Build history of the part. All positions in model axes, mm. A direction names the side the tool comes from. Give positions to 0.01 mm unless a question says otherwise; leave off trailing zeros. Loops run counter-clockwise (first coordinate to the right, second up) from the corner with the lowest first, then second, coordinate; pieces in that order, holes last. Notation, with made-up numbers: M 81.5,-21 L 138.5,-21 A24 ccw 138.5,3 Z; hole C -5,-36 d11. An arc over 180 degrees is marked long. Put each result on its own line as item: value.
```python
from build123d import *

# Parameters (mm, degrees)
SKETCH1_R                                    = 1.93
BOSS_EXTRUDE1_DEPTH                          = 7.3
BOSS_EXTRUDE2_DEPTH                          = 30
BOSS_EXTRUDE5_START                          = 15.4
SKETCH1_7_R                                  = 4
SKETCH1_7_R_2                                = 1.93
BOSS_EXTRUDE5_DEPTH                          = 7.3
CSK_FOR_M5_COUNTERSUNK_FLAT_HEAD_SCR_2_COUNT = 2
CSK_FOR_M5_COUNTERSUNK_FLAT_HEAD_SCR_2_PITCH = 15


with BuildPart() as part:
    # Sketch1 → Boss-Extrude1 (new body)
    with BuildSketch(Plane(origin=(0, 0, 0), x_dir=(1, 0, 0), z_dir=(0, 1, 0))):
        with BuildLine():
            Line((0, 4), (0, 4.45))
            Line((0, 4.45), (-18.73, 4.45))
            Line((-18.73, 4.45), (-15.127118856, 0.847118856))
            ThreePointArc((-15.127118856, 0.847118856), (-14.188807149, 0.220159018), (-13.081993025, 0))
            Line((-13.081993025, 0), (-4, 0))
            ThreePointArc((-4, 0), (2.828427125, -2.828427125), (0, 4))
        make_face()
        Circle(SKETCH1_R, mode=Mode.SUBTRACT)
    extrude(amount=BOSS_EXTRUDE1_DEPTH)

    # Sketch1_3 → Boss-Extrude2 (add)
    with BuildSketch(Plane(origin=(0, 0, 0), x_dir=(1, 0, 0), z_dir=(0, 1, 0))):
        with BuildLine():
            Line((0, 4), (0, 4.45))
            Line((0, 4.45), (-18.73, 4.45))
            Line((-18.73, 4.45), (-15.127118856, 0.847118856))
            ThreePointArc((-15.127118856, 0.847118856), (-14.188807149, 0.220159018), (-13.081993025, 0))
            Line((-13.081993025, 0), (-4, 0))
            ThreePointArc((-4, 0), (-2.828427125, 2.828427125), (0, 4))
        make_face()
    extrude(amount=BOSS_EXTRUDE2_DEPTH)

    # Sketch1_7 → Boss-Extrude5 (add)
    with BuildSketch(Plane(origin=(0, 0, 0), x_dir=(1, 0, 0), z_dir=(0, 1, 0)).offset(BOSS_EXTRUDE5_START)):
        Circle(SKETCH1_7_R)
        Circle(SKETCH1_7_R_2, mode=Mode.SUBTRACT)
    extrude(amount=BOSS_EXTRUDE5_DEPTH)

    # Sketch3 → CSK for M5 Countersunk Flat Head Screw1 (revolve, cut)
    with BuildSketch(Plane(origin=(-9.7, 23.25, 0), x_dir=(0, -1, 0), z_dir=(1, 0, 0))):
        Polygon((0, 0), (0, 4.45), (2.65, 4.45), (2.65, 3.05), (5.2, 0.5), (5.2, 0), align=None)
    csk_for_m5_countersunk_flat_head_screw1 = revolve(axis=Axis((-9.7, 23.25, 6.35), (0, 0, -1)), mode=Mode.SUBTRACT)

    # CSK for M5 Countersunk Flat Head Scr 2: CSK for M5 Countersunk Flat Head Screw1 ×2
    with Locations(*[(0, -i * CSK_FOR_M5_COUNTERSUNK_FLAT_HEAD_SCR_2_PITCH, 0) for i in range(1, CSK_FOR_M5_COUNTERSUNK_FLAT_HEAD_SCR_2_COUNT)]):
        add(csk_for_m5_countersunk_flat_head_screw1, mode=Mode.SUBTRACT)


solid = part.part
```
Q1. Mould opens along X. For faces 1 (the conical face through (-9.82, 26.06, -2.89)), 2 (the cylindrical face through (2.734, 3.599, 2.92)), 3 (the flat face through (2, 7.3, -1)), 4 (the cylindrical face through (-11.491, 10.203, -3.74)) say: pulls with the +X half, pulls with the -X half, needs draft (parallel to the pull), parting line crosses it, or undercut.
Here are the results:
face 1: undercut
face 2: parting line crosses it
face 3: needs draft
face 4: undercut
Q2. Slice it at C-C (y = 8.25). List the corners of the cut face in (x, z).
Here are the results:
outline: M -18.73,-4.45 L -12.35,-4.45 L -12.35,-3.05 L -14.82,-0.58 A2.89 ccw -15.13,-0.85 Z; M -7.05,-4.45 L 0,-4.45 L 0,-4 A4 cw -4,0 L -4.5,0 L -4.5,-0.5 L -7.05,-3.05 Z
Q3. Probe line 1 (Y direction, x = -9.7, z = -0.35); line 2 (Y direction, x = -9.7, z = -3.25); line 3 (X direction, y = 4, z = -0.75). List the from-to ranges inside material, lowest first. Write a range as from..to.
Here are the results:
line 1: 0..3.05, 13.45..18.05, 28.45..30
line 2: 0..5.6, 10.9..20.6, 25.9..30
line 3: -15.03..-12.24, -7.16..-1.78, 1.78..3.93
Q4. Slice it at D-D (x = 1). List the corners of the cut face in (y, z).
Here are the results:
outline: M 0,-3.87 L 7.3,-3.87 L 7.3,-1.65 L 0,-1.65 Z; M 0,1.65 L 7.3,1.65 L 7.3,3.87 L 0,3.87 Z; M 15.4,-3.87 L 22.7,-3.87 L 22.7,-1.65 L 15.4,-1.65 Z; M 15.4,1.65 L 22.7,1.65 L 22.7,3.87 L 15.4,3.87 Z
Q5. Drop flat-ended pins along their axis: pin 1 Ø2.5 at (x, y) = (-9, 16) entering from +Z; pin 2 Ø4 at (y, z) = (4.5, 2.5) entering from -X; pin 3 Ø3 at (x, y) = (-9, 10) entering from +Z. Give the stop position or say it passes through.
Here are the results:
pin 1: z = 0
pin 2: x = -3.97
pin 3: z = -2.32
Q6. Slice it at B-B (z = -1.5). List the corners of the cut face in (x, y).
Here are the results:
outline: M -15.78,0 L -1.21,0 L -1.21,7.3 L -3.71,7.3 L -3.71,15.4 L -1.21,15.4 L -1.21,22.7 L -3.71,22.7 L -3.71,30 L -15.78,30 Z; M 1.21,0 L 3.71,0 L 3.71,7.3 L 1.21,7.3 Z; M 1.21,15.4 L 3.71,15.4 L 3.71,22.7 L 1.21,22.7 Z; hole C -9.7,8.25 d8.4; hole C -9.7,23.25 d8.4
Q7. Slice it at A-A (x = -9.7). List the corners of the cut face in (y, z), and give its area (3 significant figures).
Here are the results:
outline: M 0,-4.45 L 5.6,-4.45 L 5.6,-3.05 L 3.05,-0.5 L 3.05,0 L 0,0 Z; M 10.9,-4.45 L 20.6,-4.45 L 20.6,-3.05 L 18.05,-0.5 L 18.05,0 L 13.45,0 L 13.45,-0.5 L 10.9,-3.05 Z; M 25.9,-4.45 L 30,-4.45 L 30,0 L 28.45,0 L 28.45,-0.5 L 25.9,-3.05 Z
area: 68.2 mm²
Q8. Tool access for faces 5 (the flat face through (-9, 30, -3)), 6 (the flat face through (2, 22.7, -1)), 7 (the cylindrical face through (-4.504, 8.459, -0.247)), 8 (the flat face through (-8, 15, 0)), 9 (the cylindrical face through (-2.859, 11.293, -2.797)): list every direction of +Z, -Z, +X, -X, +Y, -Y with a clear straight run to the whole face (end or side of a thin tool).
Here are the results:
face 5: +Z, -Z, +X, -X, +Y
face 6: +Z, +X, +Y
face 7: +Z
face 8: +Z, -X, +Y, -Y
face 9: +Z, +X
